Input: part model. Units: mm. Frame: model coordinates. Round coordinates to 2 decimals unless told otherwise and drop trailing zeros. Loops run counter-clockwise (first coordinate to the right, second up) from the corner with the lowest first, then second, coordinate; pieces in that order, holes last. Notation, with made-up numbers: M 70.5,36.5 L 82.5,36.5 A9 cw 82.5,48.5 Z; hole C -33,57 d11. An arc over 180 degrees is marked long. Return JSON: item names as keys, results as strings. Group by question number.
1) Mould query, pull axis Y, two halves, no side actions, for faces 1 (the face through (0, 30, 4.762)), 2 (the face through (49.844, 9.947, 2.161)), 3 (the face through (37.95, 0.09, 2.35)), 4 (the face through (20, -10, 2)). Classes: +Y half, -Y half, draft (parallel to the pull), parting line (faces both ways), or undercut.
2) Section C-C (y = 0). Count the separate pieces of the cut face and the enclosed holes in it, plus the area to 3 significant figures.
3) Contact query for flat-ended pins moving along their axis: P1, Ø1.5, axis at x = 10.5, z = 3, coming from the +Y side; P2, Ø10, axis at x = 41, y = 22, coming from the +Z side. Output: stop coordinate, or through.
4) Section D-D (z = 2.05). Output: boundary loops of the cut face in (x, y).
5) Material intervals for line 1 (Y direction, x = 0, z = 2.4); line 2 (Z direction, x = 11, y = 30.5); line 3 (Y direction, x = 1, z = 2.2), sorted ascending. Write a range as from..to.
from build123d import *

# Parameters (mm, degrees)
F2_W     = 6.975
F2_H     = 40
F2_H_2   = 6.975
F2_W_2   = 6.05
F2_R     = 2.05
F2_H_3   = 6.05
F2_W_3   = 40
F3_DEPTH = 4.2625
F4_DEPTH = 4.7625
F5_R     = 2


with BuildPart() as f3:
    # F2 (on Top) → F3 (new body)
    with BuildSketch(Plane.XY):
        with Locations((-6.5125, 30)):
            Rectangle(F2_W, F2_H)
        with Locations((-6.5125, 6.5125)):
            Rectangle(F2_W, F2_H_2)
        with Locations((0, 30)):
            Rectangle(F2_W_2, F2_H)
        with Locations((0, 20)):
            Circle(F2_R, mode=Mode.SUBTRACT)
        with Locations((0, 40)):
            Circle(F2_R, mode=Mode.SUBTRACT)
        with Locations((-6.5125, 0)):
            Rectangle(F2_W, F2_H_3)
        with Locations((6.5125, 30)):
            Rectangle(F2_W, F2_H)
        with Locations((-6.5125, -6.5125)):
            Rectangle(F2_W, F2_H_2)
        Polygon((50, 10), (10, 50), (10, 10), align=None)
        with Locations((0, -6.5125)):
            Rectangle(F2_W_2, F2_H_2)
        with Locations((30, 6.5125)):
            Rectangle(F2_W_3, F2_H_2)
        with Locations((6.5125, -6.5125)):
            Rectangle(F2_W, F2_H_2)
        with Locations((30, 0)):
            Rectangle(F2_W_3, F2_H_3)
        with Locations((20, 0)):
            Circle(F2_R, mode=Mode.SUBTRACT)
        with Locations((40, 0)):
            Circle(F2_R, mode=Mode.SUBTRACT)
        with Locations((30, -6.5125)):
            Rectangle(F2_W_3, F2_H_2)
        with Locations((6.5125, 6.5125)):
            Rectangle(F2_W, F2_H_2)
        with Locations((6.5125, 0)):
            Rectangle(F2_W, F2_H_3)
        Rectangle(F2_W_2, F2_H_3)
        Circle(F2_R, mode=Mode.SUBTRACT)
        with Locations((0, 6.5125)):
            Rectangle(F2_W_2, F2_H_2)
    extrude(amount=F3_DEPTH)

    # F2 (on Top) → F4 (join)
    with BuildSketch(Plane.XY):
        Rectangle(F2_W_2, F2_H_3)
        Circle(F2_R, mode=Mode.SUBTRACT)
        with Locations((30, 0)):
            Rectangle(F2_W_3, F2_H_3)
        with Locations((20, 0)):
            Circle(F2_R, mode=Mode.SUBTRACT)
        with Locations((40, 0)):
            Circle(F2_R, mode=Mode.SUBTRACT)
        with Locations((0, 30)):
            Rectangle(F2_W_2, F2_H)
        with Locations((0, 20)):
            Circle(F2_R, mode=Mode.SUBTRACT)
        with Locations((0, 40)):
            Circle(F2_R, mode=Mode.SUBTRACT)
    extrude(amount=F4_DEPTH)

    # F5
    f5_edges = [f3.edges().sort_by_distance(p)[0] for p in [
        (50, 10, 2.13125),
        (50, -10, 2.13125),
        (-10, -10, 2.13125),
        (-10, 50, 2.13125),
        (10, 50, 2.13125),
    ]]
    fillet(f5_edges, radius=F5_R)


solid = f3.part
Returned:
{
 "1": {"face 1": "draft", "face 2": "+Y half", "face 3": "undercut", "face 4": "-Y half"},
 "2": {"separate pieces": "4", "enclosed holes": "0", "area": "220 mm^2"},
 "3": {"P1": "stops at y = 49.91", "P2": "stops at z = 4.26"},
 "4": {"outline": "M -10,-8 A2 ccw -8,-10 L 48,-10 A2 ccw 50,-8 L 50,9.17 A2 ccw 49.41,10.59 L 10.59,49.41 A2 ccw 9.17,50 L -8,50 A2 ccw -10,48 Z; hole C 0,0 d4.1; hole C 0,20 d4.1; hole C 0,40 d4.1; hole C 20,0 d4.1; hole C 40,0 d4.1"},
 "5": {"line 1": "y = -10..-2.05, 2.05..17.95, 22.05..37.95, 42.05..50", "line 2": "z = 0..4.26", "line 3": "y = -10..-1.79, 1.79..18.21, 21.79..38.21, 41.79..50"}
}
